Autodesk Inventor part; units mm, degrees
ref_plane "YZ Plane" through (0, 0, 0) normal (1, 0, 0) x (0, 1, 0)
ref_plane "XZ Plane" through (0, 0, 0) normal (0, 1, 0) x (-1, 0, 0)
ref_plane "XY Plane" through (0, 0, 0) normal (0, 0, 1) x (1, 0, 0)
sketch "스케치1" plane through (0, 0, 0) normal (0, 0, 1) x (1, 0, 0)
  line L0 (-10, -5) -> (10, -5)
  line L1 (10, -5) -> (10, 5)
  line L2 (10, 5) -> (-10, 5)
  line L3 (-10, 5) -> (-10, -5)
  line L4 (-10, -5) -> (10, 5) construction
  line L5 (10, -5) -> (-10, 5) construction
  circle A0 centre (-5, 0) radius 1.5
  circle A1 centre (5, 0) radius 1.5
  point P0 (0, 0)
  dimension "d0" = 10
  dimension "d1" = 20
  dimension "d2" = 3
  dimension "d3" = 5
  dimension "d4" = 5
extrude "돌출1" add sketch "스케치1" along normal blind 10
fillet "모깎기1" radius 2 4 edges at (-10, 5, 5) (-10, -5, 5) (10, -5, 5) (10, 5, 5)
chamfer "모따기1" distance 1 angle 45 16 edges at (0, 5, 0) (-9.4142, 4.4142, 0) (-10, 0, 0) (-9.4142, -4.4142, 0) (0, -5, 0) (9.4142, -4.4142, 0) (10, 0, 0) (9.4142, 4.4142, 0) (0, 5, 10) (-9.4142, 4.4142, 10) (-10, 0, 10) (-9.4142, -4.4142, 10) (0, -5, 10) (9.4142, -4.4142, 10) (10, 0, 10) (9.4142, 4.4142, 10)
properties part number "RobotBaseConnector1x2_3D 인쇄"
Geometry: final body of the model. Coordinates: model frame, mm. Round coordinates to 2 decimals unless told otherwise and drop trailing zeros. Order: outer loops, then holes, each group sorted by start corner. A loop starts at its lowest first (then second) coordinate and runs counter-clockwise, first axis right, second up.
Q1. Section C-C, the plane x = -5. Output: boundary loops of the cut face in (y, z).
Result sheet:
outline: (-5, 1) - (-4, 0) - (-1.5, 0) - (-1.5, 10) - (-4, 10) - (-5, 9) - close; (1.5, 0) - (4, 0) - (5, 1) - (5, 9) - (4, 10) - (1.5, 10) - close
Q2. Section A-A, the plane y = 0. Output: boundary loops of the cut face in (x, z), and give its area (3 significant figures).
Result sheet:
outline: (-10, 1) - (-9, 0) - (-6.5, 0) - (-6.5, 10) - (-9, 10) - (-10, 9) - close; (-3.5, 0) - (3.5, 0) - (3.5, 10) - (-3.5, 10) - close; (6.5, 0) - (9, 0) - (10, 1) - (10, 9) - (9, 10) - (6.5, 10) - close
area: 138 mm2
Q3. Section D-D, the plane x = 0. Output: boundary loops of the cut face in (y, z).
Result sheet:
outline: (-5, 1) - (-4, 0) - (4, 0) - (5, 1) - (5, 9) - (4, 10) - (-4, 10) - (-5, 9) - close
Q4. Section B-B, the plane z = 1.75. Output: boundary loops of the cut face in (x, y).
Result sheet:
outline: (-10, -3) arc R2 ccw to (-8, -5) - (8, -5) arc R2 ccw to (10, -3) - (10, 3) arc R2 ccw to (8, 5) - (-8, 5) arc R2 ccw to (-10, 3) - close; hole circle Ø3 at (-5, 0); hole circle Ø3 at (5, 0)
Q5. Pin query (flat end, axial travel): pin 1 (2.5 mm diameter, centred on x = -5, y = 0, fed in from -Z); pin 2 (3 mm diameter, centred on x = 4.5, y = 3, fed in from -Z). Return the tip coordinate at first contact, or that it passes through.
Result sheet:
pin 1: passes through
pin 2: stops at z = 0
Q6. Mould query, pull axis X, two halves, no side actions, for faces 1 (the face through (6.386, 0.575, 4.93)), 2 (the face through (0, 0, 0)), 3 (the face through (9, -3.98, 9.6)). Classes: released by +X, released by -X, zero draft, split by the parting line, or undercut.
Result sheet:
face 1: undercut
face 2: zero draft
face 3: released by +X
Q7. Material intervals for probe 1 along Y at (x, z) = (5, 3.75); probe 2 along X at (y, z) = (0.75, 4.25); probe 3 along Y at (x, z) = (6, 5.5), sorted ascending.
Result sheet:
probe 1: y = -5 to -1.5, 1.5 to 5
probe 2: x = -10 to -6.3, -3.7 to 3.7, 6.3 to 10
probe 3: y = -5 to -1.12, 1.12 to 5
